```python
from build123d import *

# Parameters (mm, degrees)
ESQUISSE2_R             = 3
BOSS_EXTRU_1_DEPTH      = 90
ESQUISSE3_W             = 8
ESQUISSE3_H             = 8
BOSS_EXTRU_2_DEPTH      = 50
ESQUISSE8_R             = 2
ENL_V_MAT_EXTRU_4_DEPTH = 10


with BuildPart() as part:
    # Esquisse1 → Révolution1 (revolve)
    with BuildSketch(Plane.XY, mode=Mode.PRIVATE) as r_volution1_sk:
        Polygon((0, 0), (3, 0), (0, 6), align=None)
    revolve(r_volution1_sk.sketch.rotate(Axis((0, 0, 0), (0, 1, 0)), 90), axis=Axis((0, 0, 0), (0, 1, 0)))

    # Esquisse2 → Boss.-Extru.1 (add)
    with BuildSketch(Plane.XZ):
        with Locations(Location((0, 0, 0), (0, 0, 90))):
            Circle(ESQUISSE2_R)
    extrude(amount=BOSS_EXTRU_1_DEPTH)

    # Esquisse3 → Boss.-Extru.2 (add)
    with BuildSketch(Plane.XZ.offset(90)):
        Rectangle(ESQUISSE3_W, ESQUISSE3_H)
    extrude(amount=-BOSS_EXTRU_2_DEPTH)

    # Esquisse8 → Enlèv. mat.-Extru.4 (cut)
    with BuildSketch(Plane(origin=(0, 0, -4), x_dir=(-1, 0, 0), z_dir=(0, 0, -1))):
        with Locations((0, -81.574730925)):
            Circle(ESQUISSE8_R)
    extrude(amount=-ENL_V_MAT_EXTRU_4_DEPTH, mode=Mode.SUBTRACT)


solid = part.part
```
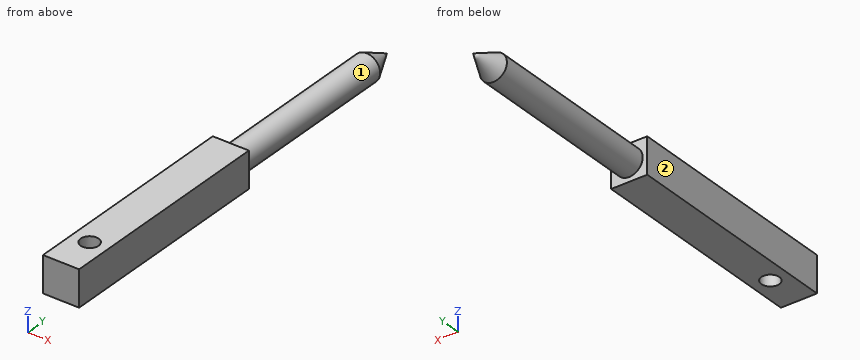
Here's how the part is built. I have some questions about the finished solid (model axes, mm). Face numbers are marked on the shaded views. A direction names the side the tool comes from. Coordinates: 2 decimals unless noted, no trailing zeros. Loops run counter-clockwise (first coordinate to the right, second up) from the corner with the lowest first, then second, coordinate; pieces in that order, holes last. Notation, with made-up numbers: (88.25, 51.25) -> (94.25, 51.25) arc R24 ccw to (94.25, 74.25) -> close; hole circle Ø7 at (-34.5, 23.5). An arc over 180 degrees is marked (long way). Return JSON: item names as keys, results as strings.
1) Will these pins go through, and if not, where does the flat tip stop? pin 1 (3 mm diameter, centred on x = 0, y = -81.57, fed in from -Z); pin 2 (2.5 mm diameter, centred on x = 0.5, z = 1.5, fed in from +Y); pin 3 (1.5 mm diameter, centred on y = -27, z = -3, fed in from +X).
Results below:
{"pin 1": "through", "pin 2": "y = 5.34", "pin 3": "x = 1.98"}
2) If we section it at A-A, the plane y = -12: Write out the boundary of the cut face in (x, z).
Results below:
{"outline": "circle Ø6 at (0, 0)"}
3) I need wall thicknesses on line 1 (Y direction, x = 0, z = 1); line 2 (Y direction, x = 0, z = 1.5); line 3 (Y direction, x = -3.5, z = 0.5). Which ranges of each line are inside material? Lowest first, please. Write a range as from..to.
Results below:
{"line 1": "-90..-83.57, -79.57..4", "line 2": "-90..-83.57, -79.57..3", "line 3": "-90..-40"}
4) For the marked faces 1 and 2, which set-ups out of +Z, -Z, +X, -X, +Y, -Y let a thin tool reach every point of the face, with its end or its side?
Results below:
{"face 1": "+Y", "face 2": "+Z, -Z, -X, +Y, -Y"}
